from build123d import *

# Parameters (mm, degrees)
CHAMFER1_SIZE = 0.5


with BuildPart() as part:
    # Sketch1 → Revolve1 (revolve)
    with BuildSketch(Plane.XY, mode=Mode.PRIVATE) as revolve1_sk:
        with BuildLine():
            Line((0, 0), (0, 7))
            Line((0, 7), (2, 7))
            Line((2, 7), (2, 6.4))
            Line((2, 6.4), (3, 6.4))
            Line((3, 6.4), (3, 7))
            Line((3, 7), (3.98, 7))
            ThreePointArc((3.98, 7), (3.948276406, 6.742305898), (3.855, 6.5))
            ThreePointArc((3.855, 6.5), (3.761723594, 6.257694102), (3.73, 6))
            Line((3.73, 6), (3.73, 0))
            Line((3.73, 0), (0, 0))
        make_face()
    revolve(revolve1_sk.sketch.rotate(Axis((0, 0, 0), (1, 0, 0)), 90), axis=Axis((0, 0, 0), (1, 0, 0)))

    # Chamfer1
    chamfer1_edges = [part.edges().sort_by_distance(p)[0] for p in [
        (0, 0, -7),
    ]]
    chamfer(chamfer1_edges, length=CHAMFER1_SIZE)


solid = part.part
Geometry check sheet. Reference: the model listing, model coordinates, mm. A direction names the side the tool comes from. Round coordinates to 2 decimals unless told otherwise and drop trailing zeros. Loops run counter-clockwise (first coordinate to the right, second up) from the corner with the lowest first, then second, coordinate; pieces in that order, holes last. Notation, with made-up numbers: (-32, 80.25) -> (-19, 80.25) arc R20 cw to (-19, 106.25) -> close; hole circle Ø7 at (-2.75, 10.5). An arc over 180 degrees is marked (long way). Answer as a JSON object with one key per item and string values. Group by question number.
Item 1: Set-up check for faces 4 (the face through (2, 6, 3)), 5 (the face through (0, 0, 0)): record each of +Z, -Z, +X, -X, +Y, -Y from which the full face is reachable in a straight line by a thin tool's end or side.
Item 2: Thickness scan on line 1 along X through (y, z) = (-2, -1.5); line 2 along X through (y, z) = (5.25, 4); line 3 along Z through (x, y) = (0.4, 5.75). Record the ranges inside material, lowest first.
Item 3: Cross-section at B-B, the plane x = 3.45. Record the cut outline in (y, z).
Item 4: Cross-section at A-A, the plane x = 2.65. Record the cut outline in (y, z).
Item 5: Release check for a two-part mould opening along X. For faces 1 (the face through (3.73, 0, 0)), 2 (the face through (3.5, 6.21, 3.23)), 3 (the face through (3, 6, -3)) record: pulls with the +X half, pulls with the -X half, needs draft (parallel to the pull), parting line crosses it, or undercut.
Item 6: Depth check by flat-ended pin: pin 1 Ø4 at (y, z) = (-1, 4.5) entering from +X; pin 2 Ø1 at (x, z) = (1, -3.5) entering from +Y; pin 3 Ø3.5 at (y, z) = (2.5, 2.5) entering from +X. Enter the tip coordinate at first touch or a pass-through.
Determined:
{
 "1": {"face 4": "none", "face 5": "+Z, -Z, -X, +Y, -Y"},
 "2": {"line 1": "x = 0 to 3.73", "line 2": "x = 0.1 to 2, 3 to 3.9", "line 3": "z = -3.81 to 3.81"},
 "3": {"outline": "circle Ø14 at (0, 0)"},
 "4": {"outline": "circle Ø12.8 at (0, 0)"},
 "5": {"face 1": "pulls with the +X half", "face 2": "needs draft", "face 3": "undercut"},
 "6": {"pin 1": "stops at x = 3.91", "pin 2": "stops at y = 6.32", "pin 3": "stops at x = 3.73"}
}
